from build123d import *

# Parameters (mm, degrees)
SKETCH1_W           = 200
SKETCH1_H           = 240
BOSS_EXTRUDE3_DEPTH = 25
SKETCH3_W           = 87.5
SKETCH3_H           = 110
CUT_EXTRUDE1_DEPTH  = 25
SKETCH4_W           = 200
SKETCH4_H           = 30.164162566
BOSS_EXTRUDE4_DEPTH = 25
FILLET4_R           = 10
FILLET5_R           = 10
SKETCH6_W           = 32
SKETCH6_H           = 30
CUT_EXTRUDE2_DEPTH  = 12.5
FILLET6_R           = 2.5
FILLET7_R           = 2.5
FILLET8_R           = 2.5
SKETCH8_W           = 72.718372575
SKETCH8_H           = 10
BOSS_EXTRUDE5_DEPTH = 40
FILLET9_R           = 2.5
CUT_EXTRUDE3_DEPTH  = 40
CUT_EXTRUDE4_DEPTH  = 40


with BuildPart() as part:
    # Sketch1 → Boss-Extrude3 (new body)
    with BuildSketch(Plane.XY):
        Rectangle(SKETCH1_W, SKETCH1_H)
    extrude(amount=BOSS_EXTRUDE3_DEPTH)

    # Sketch3 → Cut-Extrude1 (cut)
    with BuildSketch(Plane.XY.offset(25)):
        with Locations((-43.75, -55)):
            Rectangle(SKETCH3_W, SKETCH3_H)
    extrude(amount=-CUT_EXTRUDE1_DEPTH, mode=Mode.SUBTRACT)

    # Sketch4 → Boss-Extrude4 (add)
    with BuildSketch(Plane.XY.offset(25)):
        with Locations((0, -135.082081283)):
            Rectangle(SKETCH4_W, SKETCH4_H)
    extrude(amount=-BOSS_EXTRUDE4_DEPTH)

    # Fillet4
    fillet4_edges = [part.edges().sort_by_distance(p)[0] for p in [
        (-87.5, -55, 25),
    ]]
    fillet(fillet4_edges, radius=FILLET4_R)

    # Fillet5
    fillet5_edges = [part.edges().sort_by_distance(p)[0] for p in [
        (-87.5, -55, 0),
    ]]
    fillet(fillet5_edges, radius=FILLET5_R)

    # Sketch6 → Cut-Extrude2 (cut)
    with BuildSketch(Plane.XY.offset(25)):
        with Locations((-71.5, -125)):
            Rectangle(SKETCH6_W, SKETCH6_H)
    cut_extrude2 = extrude(amount=-CUT_EXTRUDE2_DEPTH, mode=Mode.SUBTRACT)

    # Fillet6
    fillet6_edges = [part.edges().sort_by_distance(p)[0] for p in [
        (-87.5, -125, 25),
    ]]
    fillet(fillet6_edges, radius=FILLET6_R)

    # Fillet7
    fillet7_edges = [part.edges().sort_by_distance(p)[0] for p in [
        (-55.5, -125, 25),
    ]]
    fillet(fillet7_edges, radius=FILLET7_R)

    # Fillet8
    fillet8_edges = [part.edges().sort_by_distance(p)[0] for p in [
        (100, -150.164162566, 12.5),
    ]]
    fillet(fillet8_edges, radius=FILLET8_R)

    # Mirror1: Cut-Extrude2 across plane
    add(cut_extrude2.mirror(Plane.ZX.offset(-55)), mode=Mode.SUBTRACT)

    # Sketch8 → Boss-Extrude5 (add)
    with BuildSketch(Plane(origin=(0, 0, 0), x_dir=(-1, 0, 0), z_dir=(0, 0, -1))):
        with Locations((-53.00826824, -68.393983819)):
            Rectangle(SKETCH8_W, SKETCH8_H)
    extrude(amount=BOSS_EXTRUDE5_DEPTH)

    # Fillet9
    fillet9_edges = [part.edges().sort_by_distance(p)[0] for p in [
        (-87.5, 15, 25),
        (-55.5, 15, 25),
    ]]
    fillet(fillet9_edges, radius=FILLET9_R)

    # Sketch9 → Cut-Extrude3 (cut)
    with BuildSketch(Plane(origin=(0, 0, 0), x_dir=(-1, 0, 0), z_dir=(0, 0, -1))):
        with BuildLine():
            Line((-91.597538887, -42.469319431), (-91.597538887, -61.749189722))
            ThreePointArc((-91.597538887, -61.749189722), (-94.256831341, -64.408482175), (-96.916123795, -61.749189722))
            Line((-96.916123795, -61.749189722), (-96.916123795, -42.469319431))
            ThreePointArc((-96.916123795, -42.469319431), (-94.256831341, -39.810026977), (-91.597538887, -42.469319431))
        make_face()
    extrude(amount=-CUT_EXTRUDE3_DEPTH, mode=Mode.SUBTRACT)

    # Sketch10 → Cut-Extrude4 (cut)
    with BuildSketch(Plane(origin=(0, 0, 0), x_dir=(-1, 0, 0), z_dir=(0, 0, -1))):
        with BuildLine():
            Line((-75.267088852, -123.445469049), (-41.491938711, -123.445469049))
            ThreePointArc((-41.491938711, -123.445469049), (-38.991938711, -125.945469049), (-41.491938711, -128.445469049))
            Line((-41.491938711, -128.445469049), (-75.267088852, -128.445469049))
            ThreePointArc((-75.267088852, -128.445469049), (-77.767088852, -125.945469049), (-75.267088852, -123.445469049))
        make_face()
    extrude(amount=-CUT_EXTRUDE4_DEPTH, mode=Mode.SUBTRACT)


solid = part.part
CAD build for the part. Positions are in the model's coordinates, mm. A direction names the side the tool comes from. Give positions to 0.01 mm unless a question says otherwise; leave off trailing zeros. Order: outer loops, then holes, each group sorted by start corner. A loop starts at its lowest first (then second) coordinate and runs counter-clockwise, first axis right, second up. Notation, with made-up numbers: (50.5, 54) - (61.5, 54) arc R31 ccw to (61.5, 86) - close; hole circle Ø5 at (66.25, 43). An arc over 180 degrees is marked (long way). Write each question's results on one line, items separated by ' | '.
1. Saw through at B-B on y = -3. List the corners of the cut face in (x, z), and give its area (3 significant figures).
Calculated:
outline: (-100, 0) - (-97.5, 0) arc R10 ccw to (-87.5, 10) - (-87.5, 15) arc R10 ccw to (-97.5, 25) - (-100, 25) - close; (0, 0) - (100, 0) - (100, 25) - (0, 25) - close | area: 2,770 mm2
2. 3-axis set-ups, long thin cutter, end or side, ignore diameter. For faces 5 (the face through (54, -63.394, -20)), 6 (the face through (89.367, -68, -20)), 7 (the face through (-72, 30, 19)), 8 (the face through (58, -128.445, 12)), 9 (the face through (-90.51, -54.23, 2.85)): which of +Z, -Z, +X, -X, +Y, -Y reach the whole face in a straight line?
Calculated:
face 5: -Z, +X, -X, +Y | face 6: -Z, +X, +Y, -Y | face 7: +Z | face 8: +Z, -Z | face 9: -Z
3. Saw through at D-D on z = 18. List the corners of the cut face in (x, y).
Calculated:
outline: (-100, -150.16) - (97.5, -150.16) arc R2.5 ccw to (100, -147.66) - (100, 120) - (-100, 120) - close; hole (-87.96, -110) - (-87.5, -110) - (-87.5, -140) - (-55.5, -140) - (-55.5, -110) - (0, -110) - (0, 0) - (-55.5, 0) - (-55.5, 30) - (-87.5, 30) - (-87.5, 0) - (-87.96, 0) - close; hole (41.49, -128.45) - (75.27, -128.45) arc R2.5 ccw to (75.27, -123.45) - (41.49, -123.45) arc R2.5 ccw to start; hole (91.6, -61.75) arc R2.66 ccw to (96.92, -61.75) - (96.92, -42.47) arc R2.66 ccw to (91.6, -42.47) - close
4. Pull direction Y, two halves, no side cores. Call faces 1 (the face through (94.32, -39.81, 12.32)), 2 (the face through (54, -68, -40)), 3 (the face through (-55.5, -125, 18)), 4 (the face through (-3, -150.164, 13)): released by +Y, released by -Y, zero draft, split by the parting line, or undercut.
Calculated:
face 1: undercut | face 2: zero draft | face 3: undercut | face 4: released by -Y
5. Saw through at C-C on x = -75. List the corners of the cut face in (y, z).
Calculated:
outline: (-150.16, 0) - (-110, 0) - (-110, 12.5) - (-140, 12.5) - (-140, 25) - (-150.16, 25) - close; (0, 0) - (120, 0) - (120, 25) - (30, 25) - (30, 12.5) - (0, 12.5) - close
6. Probe L1, parallel to X at y = 25.5, z = 14; L2, parallel to Y at x = -41.5, z = 13.5; L3, parallel to Y at x = 68.5, z = -10. List the from-to ranges inside material, lowest first. Write a range as from..to.
Calculated:
L1: x = -100..-87.5, -55.5..100 | L2: y = -150.16..-110, 0..120 | L3: y = -73.39..-63.39
7. Pin check, flat tips, straight feed: pin 1 (12 mm diameter, centred on x = -21.5, z = -8, fed in from +Y); pin 2 (5 mm diameter, centred on y = -66, z = -16, fed in from -X); pin 3 (20 mm diameter, centred on x = 62, z = -18, fed in from +Y); pin 4 (12 mm diameter, centred on x = 35, y = 19.5, fed in from -Z). Stop position of each tip, or through.
Calculated:
pin 1: passes through | pin 2: stops at x = 16.65 | pin 3: stops at y = -63.39 | pin 4: stops at z = 0
8. Saw through at A-A on x = -19. List the corners of the cut face in (y, z).
Calculated:
outline: (-150.16, 0) - (-110, 0) - (-110, 25) - (-150.16, 25) - close; (0, 0) - (120, 0) - (120, 25) - (0, 25) - close
